Can you work these out from the model? Positions are in its coordinate system, mm. Give positions to 0.01 mm unless a question says otherwise; leave off trailing zeros. Order: outer loops, then holes, each group sorted by start corner. A loop starts at its lowest first (then second) coordinate and runs counter-clockwise, first axis right, second up. Notation, with made-up numbers: M 36,50.25 L 41,50.25 A29 cw 41,86.25 Z; hole C 10,-39 d10. An arc over 180 degrees is marked long. Use one line per item in the form item = value. Start each with the question number.
1. I want a section at A-A, the plane z = 89.5. List the corners of the cut face in (x, y) for me (3 decimals).
2. I need wall thicknesses on L1, parallel to X at y = -2.3, z = 77; L2, parallel to X at y = -2.55, z = 13.5; L3, parallel to Y at x = 1.5, z = 52. Which ranges of each line are inside material? Lowest first, please.
3. I want a section at B-B, the plane y = -1.9. List the corners of the cut face in (x, z) for me.
4. Will this pin go through, and if not, where does the flat tip stop? P1, Ø10, axis at x = 23, z = 71.5, coming from the +Y side.
```python
from build123d import *

# Parameters (mm, degrees)
F0_W     = 31.75
F0_H     = 101.6
F1_DEPTH = 3.175
F2_SIZE  = 1.905


with BuildPart() as f1:
    # F0 (on Front) → F1 (new body)
    with BuildSketch(Plane.XZ):
        with Locations((15.875, 50.8)):
            Rectangle(F0_W, F0_H)
    extrude(amount=F1_DEPTH)

    # F2
    f2_edges = [f1.edges().sort_by_distance(p)[0] for p in [
        (0, -3.175, 50.8),
        (31.75, -3.175, 50.8),
    ]]
    chamfer(f2_edges, length=F2_SIZE)


solid = f1.part
```
Check result:
q1.outline = M 0,-1.27 L 1.905,-3.175 L 29.845,-3.175 L 31.75,-1.27 L 31.75,0 L 0,0 Z
q2.L1 = 1.03 to 30.72
q2.L2 = 1.28 to 30.47
q2.L3 = -2.77 to 0
q3.outline = M 0.63,0 L 31.12,0 L 31.12,101.6 L 0.63,101.6 Z
q4.P1 = 0
